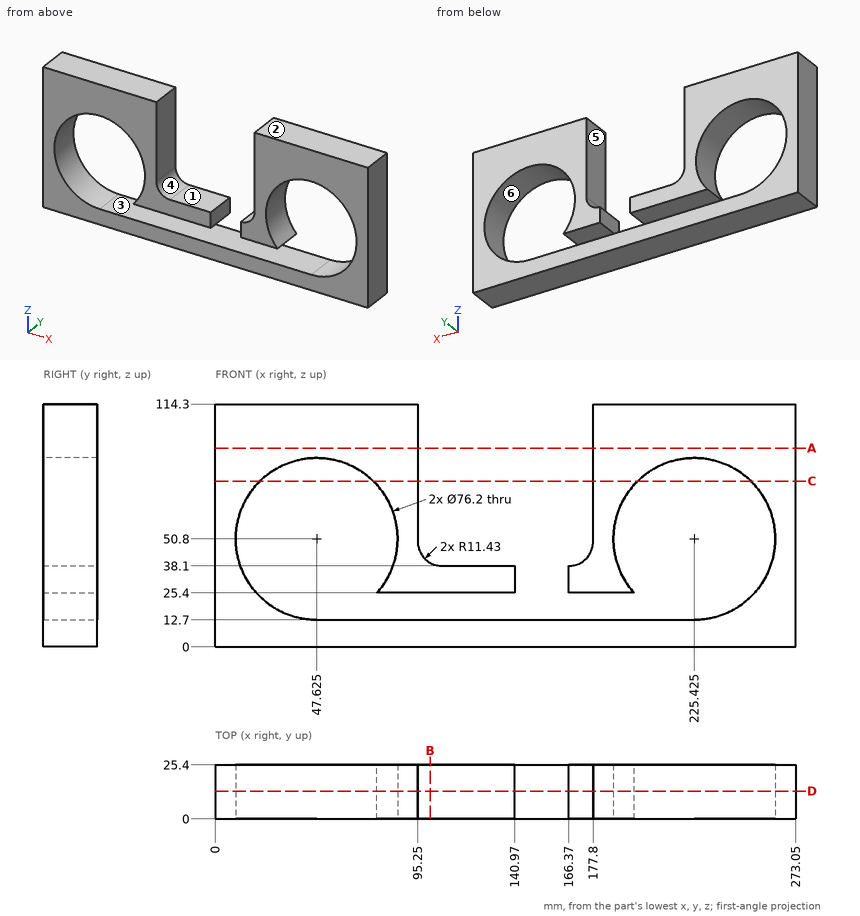
Study the drawing (mm; zero at the part's minimum x, y, z) and answer. A direction names the side the tool comes from. Coordinates: 2 decimals unless noted, no trailing zeros. Write each loop counter-clockwise with the first axis right and the second up, starting at its lowest first coordinate (ties: lowest second). Pieces come first, ordered by that corner, then holes.
Q1. Determine the mould class of the marked faces 4, 5 and 6 for opening direction Z: released by +Z, released by -Z, zero draft, split by the parting line, or undercut.
Q2. A cutting plane is placed at A-A, the plane z = 93.5. Give the vertices of the cut face in (x, y).
Q3. Each of these flat-tipped pins is pushed along its axis until it touches: pin 1 Ø10 at (x, y) = (135, 15) entering from +Z; pin 2 Ø3 at (x, y) = (150.5, 19) entering from +Z; pin 3 Ø1 at (x, y) = (231.5, 12.5) entering from -Z; pin 4 Ø6 at (x, z) = (171.5, 45.5) entering from +Y. Where does it stop, or does it pass through?
Q4. Which of the six approach directions +Z, -Z, +X, -X, +Y, -Y give full straight-line access (tool end or side, diameter ignored) to the marked faces 1, 2 and 3?
Q5. A cutting plane is placed at D-D, the plane y = 13. Give the vertices of the cut face in (x, z) (3 decimals).
Q6. Find the intervals of material crossed by line 1 (X direction, y = 11, z = 50.8) (3 decimals); line 2 (X direction, y = 9.5, z = 95); line 3 (Z direction, x = 132.5, y = 19.5), in increasing order.
Q7. A cutting plane is placed at B-B, the plane x = 101. Give the vertices of the cut face in (y, z), then the cut area to 3 significant figures.
Q8. A cutting plane is placed at C-C, the plane z = 78. Give the vertices of the cut face in (x, y).
Findings below:
1. face 4: released by +Z
1. face 5: zero draft
1. face 6: undercut
2. outline: (0, 0) - (95.25, 0) - (95.25, 25.4) - (0, 25.4) - close; (177.8, 0) - (273.05, 0) - (273.05, 25.4) - (177.8, 25.4) - close
3. pin 1: stops at z = 38.1
3. pin 2: stops at z = 12.7
3. pin 3: stops at z = 0
3. pin 4: passes through
4. face 1: +Z, +Y, -Y
4. face 2: +Z, +X, -X, +Y, -Y
4. face 3: +Y, -Y
5. outline: (0, 0) - (273.05, 0) - (273.05, 114.3) - (177.8, 114.3) - (177.8, 49.53) arc R11.43 cw to (166.37, 38.1) - (166.37, 25.4) - (197.027, 25.4) arc R38.1 cw (long way) to (225.425, 12.7) - (47.625, 12.7) arc R38.1 cw (long way) to (76.023, 25.4) - (140.97, 25.4) - (140.97, 38.1) - (106.68, 38.1) arc R11.43 cw to (95.25, 49.53) - (95.25, 114.3) - (0, 114.3) - close
6. line 1: x = 0 to 9.525, 85.725 to 95.25, 177.8 to 187.325, 263.525 to 273.05
6. line 2: x = 0 to 95.25, 177.8 to 273.05
6. line 3: z = 0 to 12.7, 25.4 to 38.1
7. outline: (0, 0) - (25.4, 0) - (25.4, 12.7) - (0, 12.7) - close; (0, 25.4) - (25.4, 25.4) - (25.4, 39.61) - (0, 39.61) - close
7. area: 684 mm2
8. outline: (0, 0) - (20.95, 0) - (20.95, 25.4) - (0, 25.4) - close; (74.3, 0) - (95.25, 0) - (95.25, 25.4) - (74.3, 25.4) - close; (177.8, 0) - (198.75, 0) - (198.75, 25.4) - (177.8, 25.4) - close; (252.1, 0) - (273.05, 0) - (273.05, 25.4) - (252.1, 25.4) - close
